Work out the finished part from the listing and answer in its coordinate system (mm). Face numbers are marked on the shaded views. Give positions to 0.01 mm unless a question says otherwise; leave off trailing zeros. Order: outer loops, then holes, each group sorted by start corner. A loop starts at its lowest first (then second) coordinate and runs counter-clockwise, first axis right, second up. Notation, with made-up numbers: (-33, 25) -> (-5, 25) arc R17 ccw to (-5, 30) -> close; hole circle Ø2 at (59.5, 13). An arc over 180 degrees is marked (long way). Answer as CSV lines item,"result". Start each with the question number.
1. For a pull along Y with two mould halves and no side action, classify the marked faces 1 and 2 as released by +Y, released by -Y, zero draft, split by the parting line, or undercut.
2. A cutting plane is placed at A-A (x = 18.5). Give the vertices of the cut face in (y, z).
3. Find the intervals of material crossed by L1, parallel to Z at x = 2, y = -1.5; L2, parallel to X at y = 2.75, z = 1.25; L3, parallel to X at y = -2.25, z = -1, in increasing order.
4. Flat-ended cylindrical pins translate along their axes: pin 1 (1 mm diameter, centred on x = 4.5, z = -0.5, fed in from +Y); pin 2 (2 mm diameter, centred on x = 20, y = -1, fed in from +Z); pin 3 (1.5 mm diameter, centred on y = 3, z = 1.5, fed in from +X). Find the tip coordinate at first contact, or state that the pin passes through.
Autodesk Inventor part; units mm, degrees
ref_plane "Work Plane1" through (29, 0, 0) normal (0, -1, 0) x (1, 0, 0)
ref_plane "YZ Plane" through (0, 0, 0) normal (1, 0, 0) x (0, 1, 0)
ref_plane "XZ Plane" through (0, 0, 0) normal (0, 1, 0) x (-1, 0, 0)
sketch "Skizze1" plane through (0, 0, 0) normal (0, 0, 1) x (1, 0, 0)
  line L0 (-0.0667, 0) -> (30, 0)
  line L1 (30, 0) -> (30, 2)
  line L2 (30, 2) -> (10, 2)
  line L3 (10, 2) -> (9.5705, 2)
  line L4 (9.5705, 2) -> (0, 2)
  line L5 (0, 2) -> (0, 3.8)
  line L6 (0, 3.8) -> (-2.2, 3.8)
  line L7 (-2.2, 3.8) -> (-2.2, 1.4434)
  line L8 (-2.2, 1.4434) -> (-0.9, 1.4434)
  line L9 (-0.9, 1.4434) -> (-0.0667, 0)
  line L10 (-8.64, 0) -> (36.44, 0)
  line L11 (0, -0.76) -> (0, 4.56)
  line L12 (10, 2) -> (0, 2) construction
  dimension "d1" = 20
  dimension "d2" = 0.4295
  dimension "d3" = 2.2
  dimension "d4" = 1.3
  dimension "d5" = 60
  dimension "d6" = 4
  dimension "d7" = 4
  dimension "d8" = 2.8868
  dimension "d9" = 7.6
  dimension "d26" = 30
revolve "Körper" add sketch "Skizze1" angle 360 about axis through (-0.0667, 0, 0) along (1, 0, 0)
sketch "Skizze2" plane through (-2.2, 0, 0) normal (-1, 0, 0) x (0, 0, 1)
  circle A0 centre (0, 0) radius 1.4434
  line L0 (0, -5.32) -> (0, 5.32)
  line L1 (-5.32, 0) -> (5.32, 0)
  line L2 (1.4434, 0) -> (0.7217, -1.25)
  line L3 (0.7217, -1.25) -> (-0.7217, -1.25)
  line L4 (-0.7217, -1.25) -> (-1.4434, 0)
  line L5 (-1.4434, 0) -> (-0.7217, 1.25)
  line L6 (-0.7217, 1.25) -> (0.7217, 1.25)
  line L7 (0.7217, 1.25) -> (1.4434, 0)
extrude "Loch" add sketch "Skizze2" against normal up to next contours L7 A0 | A0 L2 | L6 L0 A0 | A0 L0 L3 | L0 L6 A0 | A0 L3 L0 | L4 A0 | A0 L5
fillet "Rundung1" radius 1.9 1 edges at (-2.2, -3.8, 0)
thread "Gewinde"
chamfer "Fase1" distance 0.4294 distance2 0.4294 1 edges at (30, -2, 0) measured on face at (30, 0.0262, -0.4421)
ref_plane "Work Plane1" through (29, 0, 0) normal (0, -1, 0) x (1, 0, 0)
fillet "Rundung2" radius 0.2 1 edges at (0, -2, 0)
equation "\"d1\" = GEL"
equation "\"d3\" = KOH"
equation "\"d4\" = INTI"
equation "\"d6\" = GD"
equation "\"d7\" = BDM"
equation "\"d8\" = 1.1547 * SW"
equation "\"d9\" = KOD"
equation "\"d26\" = NLG"
equation "\"d17\" = RR"
equation "\"d13\" = GEL"
equation "\"d15\" = -0.5 * SPD + 0.5 * GD"
equation "\"d16\" = GUL"
equation "\"d30\" = R"
equation "\"GD\" = NND"
equation "\"NLG\" = 30"
equation "\"GEL\" = 20"
equation "\"KOD\" = 7.6"
equation "\"KOH\" = 2.2"
equation "\"INTI\" = 1.3"
equation "\"GAL\" = 0.61345 * PTC"
equation "\"GUL\" = 0.61345 * PTC"
equation "\"BDM\" = NND"
equation "\"SW\" = 2.5"
equation "\"RR\" = 1.9"
equation "\"SPD\" = NND - 1.2269 * PTC"
equation "\"R\" = 0.2"
equation "\"TOA\" = 30deg"
equation "\"GD1\" = THREADDIA - 1.2269 * PTC"
equation "\"THREADDIA\" = 4"
equation "\"PTC\" = 0.7"
equation "\"NND\" = 4"
equation "\"KOH1\" = 0.3"
equation "\"E0\" = 2.873"
properties part number "ISO 7380-1 - M4 x 30" material "Stahl"
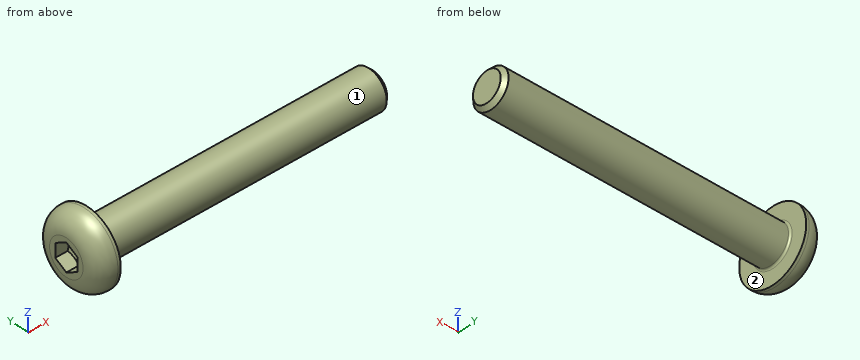
Answer sheet:
1,face 1,"split by the parting line"
1,face 2,"zero draft"
2,outline,"circle Ø4 at (0, 0)"
3,L1,"z = -1.32 to 1.32"
3,L2,"x = -1.83 to 0"
3,L3,"x = -2.11 to 0"
4,pin 1,"stops at y = 2"
4,pin 2,"stops at z = 2"
4,pin 3,"stops at x = 0"
